```python
from build123d import *

# Parameters (mm, degrees)
F0_R     = 1.6
F0_W     = 6.3
F0_H     = 1
F1_DEPTH = 3
F2_R     = 2.99999
F3_R     = 6
F4_R     = 4


# Not quite as in the source:
# - a fillet or chamfer is up to 0.001 mm smaller than in the source, because OpenCascade refuses the exact size
# - a feature names something its author has since deleted; it is built from what else it names


with BuildPart() as f1:
    # F0 (on Top) → F1 (new body)
    with BuildSketch(Plane.XY):
        with BuildLine():
            ThreePointArc((0, 3), (-2.1213203436, 2.1213203436), (-3, 0))
            Line((-3, 0), (-3, -3))
            Line((-3, -3), (-3, -4))
            Line((-3, -4), (-9.3, -4))
            Line((-9.3, -4), (-3, -14.9119200877))
            Line((-3, -14.9119200877), (3, -14.9119200877))
            Line((3, -14.9119200877), (3, -3))
            Line((3, -3), (25, -3))
            Line((25, -3), (25, 3))
            Line((25, 3), (10.0770951748, 3))
            Line((10.0770951748, 3), (7.0770951748, 3))
            Line((7.0770951748, 3), (0, 3))
        make_face()
        Circle(F0_R, mode=Mode.SUBTRACT)
        with Locations((-6.15, -3.5)):
            Rectangle(F0_W, F0_H)
        with BuildLine():
            add(Edge.make_bspline(
                [(7.0770951748, 3), (6.4332614255, 6.4067024909), (5.2223697544, 11.3722601643), (1.0114116485, 17.6559878049), (-3.6425327417, 22.6266458631), (-5, 23)],
                knots=[0, 0, 0, 0, 0.3461061531, 0.6777539699, 1, 1, 1, 1], degree=3))
            Line((7.0770951748, 3), (10.0770951748, 3))
            add(Edge.make_bspline(
                [(10.0770951748, 3), (9.3764700877, 6.6524697116), (7.4550072041, 12.4304500602), (2.9271463912, 18.7046739484), (-3.554672909, 24.5379839434), (-5, 25)],
                knots=[0, 0, 0, 0, 0.3430568532, 0.6625508471, 1, 1, 1, 1], degree=3))
            ThreePointArc((-5, 25), (-6, 24), (-5, 23))
        make_face()
    extrude(amount=F1_DEPTH)

    # F2 (radius 3 in the source; OpenCascade refuses exactly that, so slightly less here)
    f2_edges = [f1.edges().sort_by_distance(p)[0] for p in [
        (-3, -14.91192, 1.5),
        (3, -14.91192, 1.5),
        (25, -3, 1.5),
        (25, 3, 1.5),
    ]]
    fillet(f2_edges, radius=F2_R)

    # F3
    f3_edges = [f1.edges().sort_by_distance(p)[0] for p in [
        (3, -3, 1.5),
    ]]
    fillet(f3_edges, radius=F3_R)

    # F4
    f4_edges = [f1.edges().sort_by_distance(p)[0] for p in [
        (7.077095, 3, 1.5),
    ]]
    fillet(f4_edges, radius=F4_R)


solid = f1.part
```
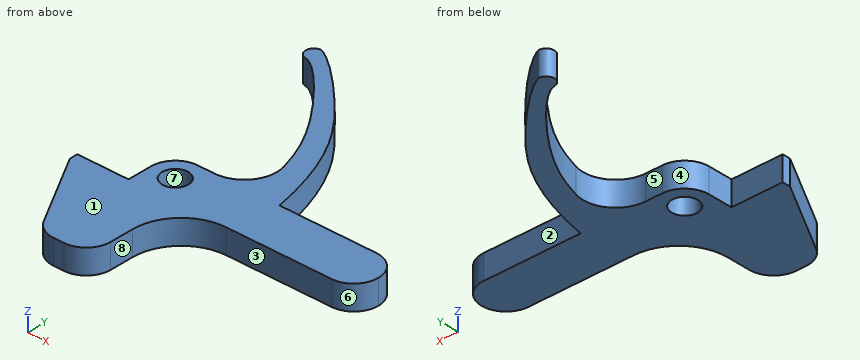
Check sheet for the modelled part. Datum: model origin and axes. Units: mm. Face numbers are marked on the shaded views. A direction names the side the tool comes from. Coordinates: 2 decimals unless noted, no trailing zeros. Loops run counter-clockwise (first coordinate to the right, second up) from the corner with the lowest first, then second, coordinate; pieces in that order, holes last.
1) Gauge pin test, flat ends, axial feed: pin 1 (0.9 mm diameter, centred on y = -1, z = 2, fed in from -X); pin 2 (1 mm diameter, centred on x = 1, z = 1, fed in from +Y); pin 3 (1.5 mm diameter, centred on x = -6, z = 1.5, fed in from +Y). Record the tip position at first contact, or that the pin passes through.
2) Sectioned sample at B-B (y = -5). Record the boundary of the cut face in (x, z), and give its area (3 significant figures).
3) Access from +Z, -Z, +X, -X, +Y, -Y to the whole of each face (thin tool, end or side, straight path). Record for the marked faces 1, 2, 3 and 4.
4) Release check for a two-part mould opening along Y. For the marked faces 5, 6, 7 and 8 record: released by +Y, released by -Y, zero draft, split by the parting line, or undercut.
5) Sectioned sample at A-A (x = 16). Record the boundary of the cut face in (y, z), and give its area (3 significant figures).
6) Material ranges on probe 1 along Y at (x, z) = (-1, 1.65); probe 2 along Y at (x, z) = (11, 2.4); probe 3 along X at (y, z) = (-2, 2.4), recorded low to high.
Check sheet entries:
1. pin 1: stops at x = -3
1. pin 2: stops at y = 20.7
1. pin 3: stops at y = 24.97
2. outline: (-8.72, 0) - (4.53, 0) - (4.53, 3) - (-8.72, 3) - close
2. area: 39.8 mm2
3. face 1: +Z, +X, -X, +Y, -Y
3. face 2: +Z, -Z, +X, +Y
3. face 3: +Z, -Z, +X, -Y
3. face 4: +Z, -Z, -X
4. face 5: undercut
4. face 6: released by -Y
4. face 7: undercut
4. face 8: zero draft
5. outline: (-3, 0) - (3, 0) - (3, 3) - (-3, 3) - close
5. area: 18.0 mm2
6. probe 1: y = -14.91 to -1.25, 1.25 to 2.83, 19.67 to 22.1
6. probe 2: y = -3 to 3
6. probe 3: x = -3 to 24.24
